Model file for the job. Use its own axes, mm. Give positions to 0.01 mm unless a question says otherwise; leave off trailing zeros. Write each loop counter-clockwise with the first axis right and the second up, starting at its lowest first coordinate (ties: lowest second). Pieces come first, ordered by that corner, then holes. Notation, with made-up numbers: (35, 18.5) - (93, 18.5) arc R20 ccw to (93, 46.5) - close; hole circle Ø6 at (0, 20). An arc over 180 degrees is marked (long way). One line per item, written item: value. Start each with the question number.
(1) Cut at C-C, the plane x = 5. List the corners of the cut face in (y, z) (3 decimals), and give its area (3 significant figures).
(2) Cut at B-B, the plane z = 1.85. List the corners of the cut face in (x, y), and give its area (3 significant figures).
(3) Probe L1, parallel to Y at x = 32, z = 2.4; L2, parallel to Y at x = 1, z = 0.75; L3, parallel to Z at x = -49.5, y = 31. List the from-to ranges inside material, lowest first.
(4) Mould opens along Y. For faces 1 (the face through (59.08, 30.58, 1.57)), 2 (the face through (7.023, 23.206, 1.565)), 3 (the face through (-3, 33, 0)) say: pulls with the +Y half, pulls with the -Y half, needs draft (parallel to the pull), parting line crosses it, or undercut.
from build123d import *

# Parameters (mm, degrees)
F0_R     = 4.6477092711
F1_DEPTH = 3.175
F2_SIZE2 = 10.15999
F2_SIZE  = 3.17499


# Not quite as in the source:
# - a fillet or chamfer is up to 0.001 mm smaller than in the source, because OpenCascade refuses the exact size


with BuildPart() as f1:
    # F0 (on Top) → F1 (new body)
    with BuildSketch(Plane.XY):
        with BuildLine():
            Line((54.7894574702, 39.7151075304), (-65.8053308725, 39.7151075304))
            Line((-65.8053308725, 39.7151075304), (-39.4252166152, 21.4519556612))
            Line((-39.4252166152, 21.4519556612), (54.7894574702, 25.0102191872))
            ThreePointArc((54.7894574702, 25.0102191872), (62.1419016418, 32.3626633588), (54.7894574702, 39.7151075304))
        make_face()
        with Locations((54.7894574702, 32.3626633588)):
            Circle(F0_R, mode=Mode.SUBTRACT)
    extrude(amount=F1_DEPTH)

    # F2 (size 3.175 and 10.16 in the source; OpenCascade refuses exactly that, so slightly less here)
    f2_edges = [f1.edges().sort_by_distance(p)[0] for p in [
        (-52.615274, 30.583532, 3.175),
    ]]
    f2_side = f1.faces().sort_by_distance((-52.615274, 30.583532, 1.5875))[0]
    chamfer(f2_edges, length=F2_SIZE, length2=F2_SIZE2, reference=f2_side)


solid = f1.part
Answers follow:
1. outline: (23.13, 0) - (39.715, 0) - (39.715, 3.175) - (23.13, 3.175) - close
1. area: 52.7 mm²
2. outline: (-55.4, 39.72) - (-29.56, 21.82) - (54.79, 25.01) arc R7.35 ccw to (54.79, 39.72) - close; hole circle Ø9.3 at (54.79, 32.36)
2. area: 1,620 mm²
3. L1: y = 24.15 to 39.72
3. L2: y = 22.98 to 39.72
3. L3: z = 0 to 0.66
4. face 1: undercut
4. face 2: pulls with the -Y half
4. face 3: needs draft
